from build123d import *

# Parameters (mm, degrees)
ESTRUSIONE_ESTRUSIONE1_DEPTH = 15
SCHIZZO2_R                   = 3
TAGLIO_ESTRUSIONE1_DEPTH     = 15
FORO_FILETTATO_M4_1_D        = 3.3


with BuildPart() as part:
    # Schizzo1 → Estrusione-Estrusione1 (new body)
    with BuildSketch(Plane.XY):
        Polygon((0, 0), (-20, 0), (-20, 30), (-12, 30), (-12, 8), (0, 8), align=None)
    extrude(amount=ESTRUSIONE_ESTRUSIONE1_DEPTH)

    # Schizzo2 → Taglio-Estrusione1 (cut)
    with BuildSketch(Plane.XZ):
        with Locations((-5, 7.5)):
            Circle(SCHIZZO2_R)
    extrude(amount=-TAGLIO_ESTRUSIONE1_DEPTH, mode=Mode.SUBTRACT)

    # Foro filettato M4-1 (through all)
    with Locations(Plane.XY.offset(15)):
        with Locations((-16, 25)):
            Hole(FORO_FILETTATO_M4_1_D / 2)


solid = part.part
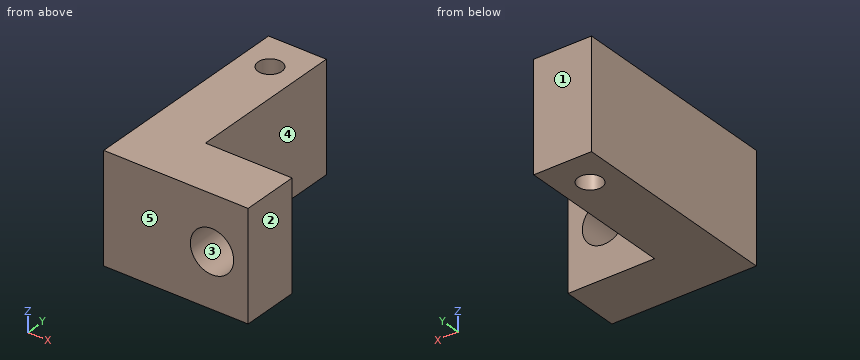
Work out the finished part from the listing and answer in its coordinate system (mm). Face numbers are marked on the shaded views. A direction names the side the tool comes from. Give positions to 0.01 mm unless a question says otherwise; leave off trailing zeros. Write each loop counter-clockwise with the first axis right and the second up, starting at its lowest first coordinate (ties: lowest second). Pieces come first, ordered by that corner, then holes. Notation, with made-up numbers: (45, -4.75) - (97, -4.75) arc R17 ccw to (97, 10.25) - close; hole circle Ø5 at (5, -1.5). An arc over 180 degrees is marked (long way). One line per item, written item: value. Start each with the question number.
1. For the marked faces 4 and 5, determine the directions among +Z, -Z, +X, -X, +Y, -Y from which every point of the face is accessible in a straight line to the end or side of a thin tool.
2. Find section D-D (y = 21.25). Write down the section's boundary in (x, z), then the cut area to 3 significant figures.
3. Consider probe 1 along Y at (x, z) = (-16, 7.5); probe 2 along Y at (x, z) = (-9.5, 6.75); probe 3 along X at (y, z) = (20.25, 3.5). Determine where each line is inside the solid, lowest interval first.
4. Find section C-C (y = 25.5). Write down the section's boundary in (x, z).
5. Given pin 1 (5 mm diameter, centred on x = -8.5, y = 26, fed in from +Z); pin 2 (3.5 mm diameter, centred on x = -8.5, z = 8, fed in from +Y); pin 3 (1 mm diameter, centred on y = 13.5, z = 9.5, fed in from +X), each flat-ended and moving along its own axis, determine where each tip first touches the part or whether it passes through.
6. Find section B-B (z = 13.5). Write down the section's boundary in (x, y).
7. For a pull along X with two mould halves and no side action, classify the marked faces 1, 2 and 3 as +X half, -X half, draft (parallel to the pull), parting line (faces both ways), or undercut.
8. Find section A-A (x = -16). Write down the section's boundary in (y, z), then the cut area to 4 significant figures.
Geometry results:
1. face 4: +Z, -Z, +X, +Y
1. face 5: +Z, -Z, +X, -X, -Y
2. outline: (-20, 0) - (-12, 0) - (-12, 15) - (-20, 15) - close
2. area: 120 mm2
3. probe 1: 0 to 23.35, 26.65 to 30
3. probe 2: 0 to 8
3. probe 3: -20 to -12
4. outline: (-20, 0) - (-17.57, 0) - (-17.57, 15) - (-20, 15) - close; (-14.43, 0) - (-12, 0) - (-12, 15) - (-14.43, 15) - close
5. pin 1: through
5. pin 2: y = 8
5. pin 3: x = -12
6. outline: (-20, 0) - (0, 0) - (0, 8) - (-12, 8) - (-12, 30) - (-20, 30) - close; hole circle Ø3.3 at (-16, 25)
7. face 1: draft
7. face 2: +X half
7. face 3: undercut
8. outline: (0, 0) - (23.35, 0) - (23.35, 15) - (0, 15) - close; (26.65, 0) - (30, 0) - (30, 15) - (26.65, 15) - close
8. area: 400.5 mm2
